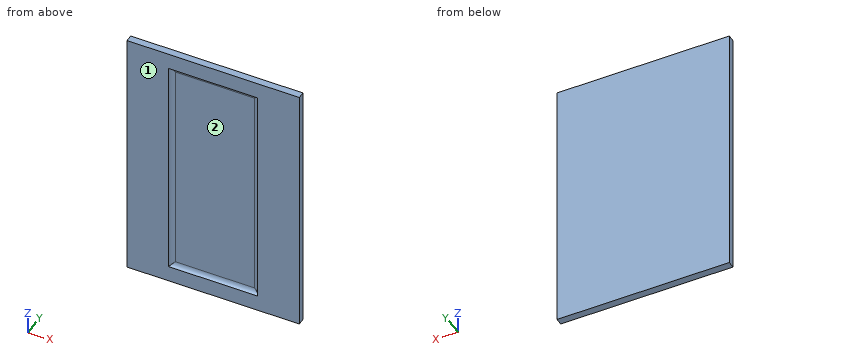
```python
from build123d import *

# Parameters (mm, degrees)
F0_W        = 304.8
F0_H        = 461.01
F1_DEPTH    = 12.7
F2_W        = 157.1649909019
F2_H        = 403.2308459282
F3_DEPTH    = 6.35
F4_T1_DEPTH = 445.8279408996
F4_T3_DEPTH = 199.7620858733


# Not quite as in the source:
# - a fillet or chamfer that OpenCascade refuses, or shapes differently, is made with other operations: its cross-section is extruded or revolved along the edge and cut away or added


with BuildPart() as f1:
    # F0 (on Front) → F1 (new body)
    with BuildSketch(Plane.XZ):
        Rectangle(F0_W, F0_H)
    extrude(amount=F1_DEPTH)

    # F2 (on face) → F3 (cut)
    with BuildSketch(Plane.XZ.offset(12.7)):
        Rectangle(F2_W, F2_H)
    extrude(amount=-F3_DEPTH, mode=Mode.SUBTRACT)

    # F4: fillet of radius 8.89 on 4 edges, made by hand

    # F4_s2 → F4_t1 (join)
    with BuildSketch(Plane.XY.offset(-222.9139704498)):
        with BuildLine():
            ThreePointArc((78.582495451, -12.7), (75.3758676252, -8.1121426782), (70.0630764567, -6.35))
            Line((70.0630764567, -6.35), (78.582495451, -6.35))
            Line((78.582495451, -6.35), (78.582495451, -12.7))
        make_face()
        with BuildLine():
            ThreePointArc((-78.582495451, -12.7), (-75.3758676252, -8.1121426782), (-70.0630764567, -6.35))
            Line((-70.0630764567, -6.35), (-78.582495451, -6.35))
            Line((-78.582495451, -6.35), (-78.582495451, -12.7))
        make_face()
    extrude(amount=F4_T1_DEPTH)

    # F4_s4 → F4_t3 (join)
    with BuildSketch(Plane.YZ.offset(-99.8810429367)):
        with BuildLine():
            ThreePointArc((-12.7, 201.6154229641), (-8.1121426782, 198.4087951383), (-6.35, 193.0960039698))
            Line((-6.35, 193.0960039698), (-6.35, 201.6154229641))
            Line((-6.35, 201.6154229641), (-12.7, 201.6154229641))
        make_face()
        with BuildLine():
            ThreePointArc((-12.7, -201.6154229641), (-8.1121426782, -198.4087951383), (-6.35, -193.0960039698))
            Line((-6.35, -193.0960039698), (-6.35, -201.6154229641))
            Line((-6.35, -201.6154229641), (-12.7, -201.6154229641))
        make_face()
    extrude(amount=F4_T3_DEPTH)


solid = f1.part
```
Check sheet for the modelled part. Datum: model origin and axes. Units: mm. Face numbers are marked on the shaded views. Round coordinates to 2 decimals unless told otherwise and drop trailing zeros. Order: outer loops, then holes, each group sorted by start corner. A loop starts at its lowest first (then second) coordinate and runs counter-clockwise, first axis right, second up. Notation, with made-up numbers: (58.5, -13.75) - (102.5, -13.75) arc R26 ccw to (102.5, 16.25) - close; hole circle Ø1 at (-11.75, -38.75). An arc over 180 degrees is marked (long way). Answer as CSV lines item,"result". Start each with the question number.
1) Draft check along X on the marked faces 1 and 2. Enter one of: +X half, -X half, draft (parallel to the pull), parting line (faces both ways), or undercut.
2) Section check C-C (y = -10.5). Record the cut outline in (x, z) (3 decimals).
3) Depth check by flat-ended pin: pin 1 (4 mm diameter, centred on x = 34, z = -151.5, fed in from -Y). Enter the tip coordinate at first touch or a pass-through.
4) Section check B-B (z = 168). Record the cut outline in (x, y), then the cut area to 3 significant figures.
5) Section check A-A (x = 10.5). Record the cut outline in (y, z) (3 decimals), then the cut area to 3 significant figures.
6) Scan lines: probe 1 along Y at (x, z) = (-21.5, -140.5); probe 2 along X at (y, z) = (-8, -95); probe 3 along X at (y, z) = (-9.5, 129). Record each from-to range of solid material in increasing order.
Determined:
1,face 1,"draft"
1,face 2,"undercut"
2,outline,"(-152.4, -230.505) - (152.4, -230.505) - (152.4, 230.505) - (-152.4, 230.505) - close; hole (-77.584, -200.617) - (77.584, -200.617) - (77.584, 200.617) - (-77.584, 200.617) - close"
3,pin 1,"y = -6.35"
4,outline,"(-152.4, -12.7) - (-78.58, -12.7) arc R8.89 cw to (-70.06, -6.35) - (70.06, -6.35) arc R8.89 cw to (78.58, -12.7) - (152.4, -12.7) - (152.4, 0) - (-152.4, 0) - close"
4,area,"2,900 mm^2"
5,outline,"(-12.7, -230.505) - (0, -230.505) - (0, 230.505) - (-12.7, 230.505) - (-12.7, 201.615) arc R8.89 cw to (-6.35, 193.096) - (-6.35, -193.096) arc R8.89 cw to (-12.7, -201.615) - close"
5,area,"3,320 mm^2"
6,probe 1,"-6.35 to 0"
6,probe 2,"-152.4 to -75.22, 75.22 to 152.4"
6,probe 3,"-152.4 to -76.85, 76.85 to 152.4"
